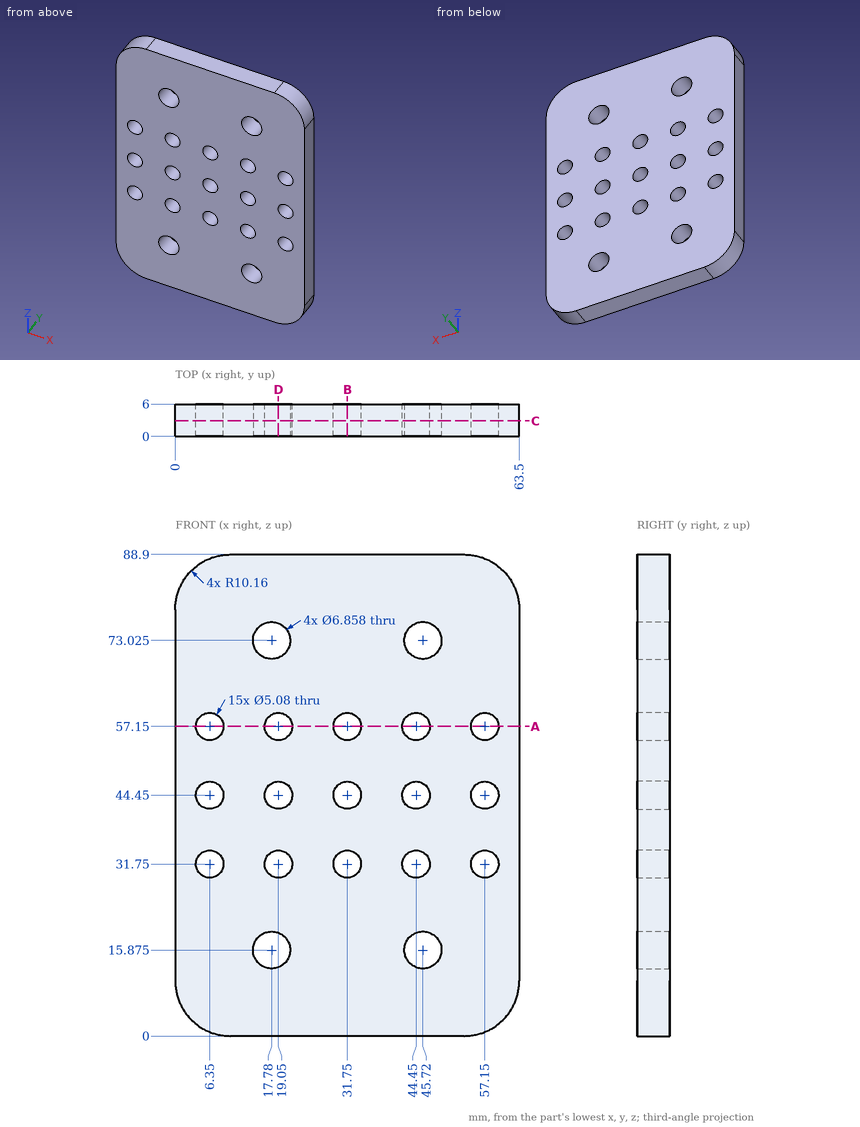
Check sheet for the drawn part. Datum: minimum x, y, z corner. Units: mm. Give positions to 0.01 mm unless a question says otherwise; leave off trailing zeros. Write each loop counter-clockwise with the first axis right and the second up, starting at its lowest first coordinate (ties: lowest second). Pieces come first, ordered by that corner, then holes.
(1) Cross-section at D-D (x = 19.05). Enter the section's corners in (y, z), plus the area to 3 significant figures.
(2) Material ranges on line 1 (X direction, y = 3.5, z = 44.45); line 2 (X direction, y = 3.65, z = 13); line 3 (X direction, y = 5.1, z = 55), recorded low to high.
(3) Cross-section at C-C (y = 2.9). State how many separate pieces and enclosed holes the cut face has, plus the area to 3 significant figures.
(4) Cross-section at A-A (z = 57.15). Enter the section's corners in (x, y), plus the area to 3 significant figures.
(5) Gauge pin test, flat ends, axial feed: pin 1 (6.5 mm diameter, centred on x = 19.05, z = 44.45, fed in from +Y); pin 2 (1.5 mm diameter, centred on x = 9, y = 3, fed in from +Z); pin 3 (4.5 mm diameter, centred on x = 6.35, z = 31.75, fed in from +Y) (3 decimals). Record the tip position at first contact, or that the pin passes through.
(6) Cross-section at B-B (x = 31.75). Enter the section's corners in (y, z), plus the area to 3 significant figures.
Worked out:
1. outline: (0, 0) - (6, 0) - (6, 12.69) - (0, 12.69) - close; (0, 19.06) - (6, 19.06) - (6, 29.21) - (0, 29.21) - close; (0, 34.29) - (6, 34.29) - (6, 41.91) - (0, 41.91) - close; (0, 46.99) - (6, 46.99) - (6, 54.61) - (0, 54.61) - close; (0, 59.69) - (6, 59.69) - (6, 69.84) - (0, 69.84) - close; (0, 76.21) - (6, 76.21) - (6, 88.9) - (0, 88.9) - close
1. area: 366 mm2
2. line 1: x = 0 to 3.81, 8.89 to 16.51, 21.59 to 29.21, 34.29 to 41.91, 46.99 to 54.61, 59.69 to 63.5
2. line 2: x = 0 to 15.91, 19.65 to 43.85, 47.59 to 63.5
2. line 3: x = 0 to 5, 7.7 to 17.7, 20.4 to 30.4, 33.1 to 43.1, 45.8 to 55.8, 58.5 to 63.5
3. separate pieces: 1
3. enclosed holes: 19
3. area: 5,100 mm2
4. outline: (0, 0) - (3.81, 0) - (3.81, 6) - (0, 6) - close; (8.89, 0) - (16.51, 0) - (16.51, 6) - (8.89, 6) - close; (21.59, 0) - (29.21, 0) - (29.21, 6) - (21.59, 6) - close; (34.29, 0) - (41.91, 0) - (41.91, 6) - (34.29, 6) - close; (46.99, 0) - (54.61, 0) - (54.61, 6) - (46.99, 6) - close; (59.69, 0) - (63.5, 0) - (63.5, 6) - (59.69, 6) - close
4. area: 229 mm2
5. pin 1: stops at y = 6
5. pin 2: stops at z = 88.89
5. pin 3: passes through
6. outline: (0, 0) - (6, 0) - (6, 29.21) - (0, 29.21) - close; (0, 34.29) - (6, 34.29) - (6, 41.91) - (0, 41.91) - close; (0, 46.99) - (6, 46.99) - (6, 54.61) - (0, 54.61) - close; (0, 59.69) - (6, 59.69) - (6, 88.9) - (0, 88.9) - close
6. area: 442 mm2
